Work out the finished part from the listing and answer in its coordinate system (mm). A direction names the side the tool comes from. Give positions to 0.01 mm unless a question says otherwise; leave off trailing zeros. Write each loop counter-clockwise with the first axis right and the second up, starting at its lowest first coordinate (ties: lowest second). Pieces come first, ordered by that corner, then holes. Notation, with made-up numbers: (57.5, 7.25) - (108.5, 7.25) arc R19 ccw to (108.5, 36.25) - close; hole circle Ø2 at (13.25, 45.5). An arc over 180 degrees is marked (long way). Write each question's results on one line, items separated by ' | '. Start each with the question number.
from build123d import *

# Parameters (mm, degrees)
F1_W     = 250.825
F1_H     = 2.54
F2_DEPTH = 57.15
F3_W     = 2.54
F3_H     = 25.4
F4_DEPTH = 302.26
F6_R     = 4
F7_DEPTH = 302.26


with BuildPart() as f2:
    # F1 (on Top) → F2 (new body)
    with BuildSketch(Plane.XY):
        with Locations((0, 1.27)):
            Rectangle(F1_W, F1_H)
        with Locations((0, 303.53)):
            Rectangle(F1_W, F1_H)
    extrude(amount=F2_DEPTH)

    # F6 (on Front) → F7 (join, through all)
    with BuildSketch(Plane.XZ):
        with Locations((40, 39.747968)):
            Circle(F6_R)
    extrude(amount=-F7_DEPTH)



with BuildPart() as f4:
    # F3 (on Front) → F4 (new body, through all)
    with BuildSketch(Plane.XZ):
        with Locations((124.1425, 12.7)):
            Rectangle(F3_W, F3_H)
    extrude(amount=-F4_DEPTH)


with BuildPart() as f5_1:
    # F5: instance of F4
    add(f4.part.mirror(Plane.YZ))


with BuildPart() as f2_1:
    add(f2.part)

    add(f4.part)  # F8 merges F4

    add(f5_1.part)  # F8 merges F5_1
    # F8: F2 across plane


with BuildPart() as f2_2:
    add(f2_1.part)
    add(f2_1.part.mirror(Plane.YZ))


solid = f2_2.part
Q1. The mould has two halves that part along Y. Classify faces 4 (the flat face through (-125.412, 150, 9)), 5 (the flat face through (-2, 0, 29)), 6 (the cylindrical face through (-39.479, 150.302, 43.714)): pulls with the +Y half, pulls with the -Y half, needs draft (parallel to the pull), parting line crosses it, or undercut.
Q2. Consider L1, parallel to Y at x = -21, z = 8; L2, parallel to X at y = 177.5, z = 13; L3, parallel to X at y = 118.5, z = 43. Determine where each line is inside the solid, lowest interval first.
Q3. Given pin 1 (3 mm diameter, centred on x = 124.5, y = 106.5, fed in from +Z), flat-ended and moving along its own axis, determine where the tip first touches the part or whether it passes through.
Q4. A cutting plane is placed at C-C, the plane x = -40. Write down the section's boundary in (y, z).
Q5. A tool of negligible diameter and unlimited length cuts with its end or side. For faces 1 (the flat face through (122.872, 150, 13)), 2 (the cylindrical face through (39.479, 150.302, 43.714)), 3 (the flat face through (-2, 304.8, 28)), from which of +Z, -Z, +X, -X, +Y, -Y can it reach the whole face along a straight path? Write none if from no direction.
Q6. A cutting plane is placed at B-B, the plane z = 7.5. Write down the section's boundary in (x, y).
Q7. A cutting plane is placed at A-A, the plane x = -70. Write down the section's boundary in (y, z).
Q8. A cutting plane is placed at D-D, the plane y = 163. Write down the section's boundary in (x, z), and give its area (3 significant figures).
Result:
1) face 4: needs draft | face 5: pulls with the -Y half | face 6: undercut
2) L1: y = 0 to 2.54, 302.26 to 304.8 | L2: x = -125.41 to -122.87, 122.87 to 125.41 | L3: x = -42.33 to -37.67, 37.67 to 42.33
3) pin 1: stops at z = 25.4
4) outline: (0, 0) - (2.54, 0) - (2.54, 35.75) - (302.26, 35.75) - (302.26, 0) - (304.8, 0) - (304.8, 57.15) - (302.26, 57.15) - (302.26, 43.75) - (2.54, 43.75) - (2.54, 57.15) - (0, 57.15) - close
5) face 1: +Z, -Z | face 2: none | face 3: +Z, -Z, +X, -X, +Y
6) outline: (-125.41, 0) - (125.41, 0) - (125.41, 304.8) - (-125.41, 304.8) - close; hole (-122.87, 2.54) - (122.87, 2.54) - (122.87, 302.26) - (-122.87, 302.26) - close
7) outline: (0, 0) - (2.54, 0) - (2.54, 57.15) - (0, 57.15) - close; (302.26, 0) - (304.8, 0) - (304.8, 57.15) - (302.26, 57.15) - close
8) outline: (-125.41, 0) - (-122.87, 0) - (-122.87, 25.4) - (-125.41, 25.4) - close; circle Ø8 at (-40, 39.75); circle Ø8 at (40, 39.75); (122.87, 0) - (125.41, 0) - (125.41, 25.4) - (122.87, 25.4) - close | area: 230 mm2
